Geometry: final body of the model. Coordinates: model frame, mm. Face numbers are marked on the shaded views. Round coordinates to 2 decimals unless told otherwise and drop trailing zeros. Write each loop counter-clockwise with the first axis right and the second up, starting at its lowest first coordinate (ties: lowest second). Pieces come first, ordered by that corner, then holes. Notation, with made-up numbers: (41, 40.5) -> (53, 40.5) arc R22 ccw to (53, 48.5) -> close; hole circle Ø2 at (14.25, -25.75). An arc over 180 degrees is marked (long way). Use one line per item in the form item = value. Start each with the question number.
1. Cut plane A-A, the plane x = 27.5. Return the cut outline in (y, z) (3 decimals).
2. Pin query (flat end, axial travel): pin 1 Ø1.5 at (y, z) = (28.5, 3) entering from -X; pin 2 Ø1.6 at (y, z) = (13.5, 3.5) entering from -X; pin 3 Ø2.5 at (x, z) = (2.5, 2.5) entering from +Y. Return the tip coordinate at first contact, or that it passes through.
3. Cut plane D-D, the plane y = 3.5. Return the cut outline in (x, z).
4. Cut plane B-B, the plane x = 7.5. Return the cut outline in (y, z) (3 decimals), plus the area to 3 significant figures.
5. Draft query along X for the marked faces 1 and 2. Return one class per face: pulls with the +X half, pulls with the -X half, needs draft (parallel to the pull), parting line crosses it, or undercut.
6. Line query: L1, parallel to Y at x = 7.5, z = 1.9 (3 decimals); L2, parallel to Y at x = 8, z = 1.85; L3, parallel to Y at x = 1, z = 3.95. Output: solid intervals per line, ascending.
7. Cut plane C-C, the plane y = 33. Return the cut outline in (x, z), plus the area to 3 significant figures.
```python
from build123d import *

# Parameters (mm, degrees)
SKETCH_1_W           = 40
SKETCH_1_H           = 25
EXTRUDE_1_DEPTH      = 5
SKETCH_2_W           = 25
SKETCH_2_H           = 62
EXTRUDE_2_DEPTH      = 5
SKETCH_3_R           = 8
CUT_EXTRUDE_1_DEPTH  = 14
EXTRUDE_3_DEPTH      = 5
EXTRUDE_4_DEPTH      = 5
SKETCH_6_R           = 1.25
CUT_EXTRUDE_2_DEPTH  = 10
SKETCH_7_R           = 13
CUT_EXTRUDE_3_DEPTH  = 10
FILLET_1_R           = 3
EXTRUDE_6_DEPTH      = 5
FILLET_5_R           = 4
SKETCH_12_R          = 15
SKETCH_12_R_2        = 8
EXTRUDE_7_DEPTH      = 5
CUT_EXTRUDE_6_DEPTH  = 10
SKETCH_14_W          = 30.1
SKETCH_14_H          = 3.1
CUT_EXTRUDE_7_DEPTH  = 5
SKETCH_15_R          = 1.05
CUT_EXTRUDE_8_DEPTH  = 5
SKETCH_18_R          = 1.5
CUT_EXTRUDE_12_DEPTH = 10
SKETCH_20_R          = 1.525
CUT_EXTRUDE_14_DEPTH = 10


with BuildPart() as part:
    # 草图1 → 凸台-拉伸1 (new body)
    with BuildSketch(Plane.XY):
        Rectangle(SKETCH_1_W, SKETCH_1_H)
    extrude(amount=EXTRUDE_1_DEPTH)

    # 草图2 → 凸台-拉伸2 (add)
    with BuildSketch(Plane.XY.offset(5)):
        with Locations((7.5, 43.5)):
            Rectangle(SKETCH_2_W, SKETCH_2_H)
    extrude(amount=-EXTRUDE_2_DEPTH)

    # 草图3 → 切除-拉伸1 (cut)
    with BuildSketch(Plane(origin=(0, 0, 0), x_dir=(-1, 0, 0), z_dir=(0, 0, -1))):
        with Locations((-7.5, 64.5)):
            Circle(SKETCH_3_R)
    extrude(amount=-CUT_EXTRUDE_1_DEPTH, mode=Mode.SUBTRACT)

    # 草图4 → 凸台-拉伸3 (add)
    with BuildSketch(Plane(origin=(0, 0, 0), x_dir=(-1, 0, 0), z_dir=(0, 0, -1))):
        Polygon((5, 74.5), (20, 12.5), (5, 12.5), align=None)
    extrude(amount=-EXTRUDE_3_DEPTH)

    # 草图5 → 凸台-拉伸4 (add)
    with BuildSketch(Plane(origin=(0, 0, 0), x_dir=(-1, 0, 0), z_dir=(0, 0, -1))):
        with BuildLine():
            Line((5, 74.5), (43.961916065, 66.994501049))
            ThreePointArc((43.961916065, 66.994501049), (66.453639267, 36.062373582), (37.102191657, 11.543673671))
            Line((37.102191657, 11.543673671), (20, 12.5))
            Line((20, 12.5), (5, 74.5))
        make_face()
    extrude(amount=-EXTRUDE_4_DEPTH)

    # 草图6 → 切除-拉伸2 (cut)
    with BuildSketch(Plane(origin=(0, 0, 0), x_dir=(-1, 0, 0), z_dir=(0, 0, -1))):
        with Locations((38.665463282, 64)):
            Circle(SKETCH_6_R)
        with Locations((59.883085674, 51.75)):
            Circle(SKETCH_6_R)
        with Locations((59.883085674, 27.25)):
            Circle(SKETCH_6_R)
        with Locations((38.665463282, 15)):
            Circle(SKETCH_6_R)
        with Locations((17.447840889, 27.25)):
            Circle(SKETCH_6_R)
        with Locations((17.447840889, 51.75)):
            Circle(SKETCH_6_R)
    extrude(amount=-CUT_EXTRUDE_2_DEPTH, mode=Mode.SUBTRACT)

    # 草图7 → 切除-拉伸3 (cut)
    with BuildSketch(Plane(origin=(0, 0, 0), x_dir=(-1, 0, 0), z_dir=(0, 0, -1))):
        with Locations((38.665463282, 39.5)):
            Circle(SKETCH_7_R)
    extrude(amount=-CUT_EXTRUDE_3_DEPTH, mode=Mode.SUBTRACT)

    # 圆角1
    fillet_1_edges = [part.edges().sort_by_distance(p)[0] for p in [
        (20, 74.5, 2.5),
        (20, -12.5, 2.5),
        (-20, -12.5, 2.5),
        (-20, 12.5, 2.5),
    ]]
    fillet(fillet_1_edges, radius=FILLET_1_R)

    # 草图9 → 凸台-拉伸6 (add)
    with BuildSketch(Plane(origin=(0, 0, 0), x_dir=(-1, 0, 0), z_dir=(0, 0, -1))):
        Polygon((-17, -12.5), (-35, -12.5), (-35, 12.5), (-19.908611993, 72.234830778), align=None)
    extrude(amount=-EXTRUDE_6_DEPTH)

    # 圆角5
    fillet_5_edges = [part.edges().sort_by_distance(p)[0] for p in [
        (35, -12.5, 2.5),
        (35, 12.5, 2.5),
    ]]
    fillet(fillet_5_edges, radius=FILLET_5_R)

    # 草图12 → 凸台-拉伸7 (add)
    with BuildSketch(Plane(origin=(0, 0, 0), x_dir=(-1, 0, 0), z_dir=(0, 0, -1))):
        with Locations((-7.5, 64.5)):
            Circle(SKETCH_12_R)
        with Locations((-7.5, 64.5)):
            Circle(SKETCH_12_R_2, mode=Mode.SUBTRACT)
    extrude(amount=-EXTRUDE_7_DEPTH)

    # 草图13 → 切除-拉伸6 (cut)
    with BuildSketch(Plane(origin=(0, 0, 0), x_dir=(-1, 0, 0), z_dir=(0, 0, -1))):
        with BuildLine():
            Line((7.401386096, 66.217175707), (7.881923771, 62.047143837))
            ThreePointArc((7.881923771, 62.047143837), (11.961869133, 57.036355872), (18.223004987, 58.633893981))
            ThreePointArc((18.223004987, 58.633893981), (30.76141934, 66.361237674), (45.486790657, 66.65638954))
            Line((45.486790657, 66.65638954), (-3.845717477, 79.048065825))
            ThreePointArc((-3.845717477, 79.048065825), (3.779900034, 74.38756063), (7.401386096, 66.217175707))
        make_face()
    extrude(amount=-CUT_EXTRUDE_6_DEPTH, mode=Mode.SUBTRACT)

    # 草图14 → 切除-拉伸7 (cut)
    with BuildSketch(Plane.XY.offset(5)):
        with Locations((7.5, 14)):
            Rectangle(SKETCH_14_W, SKETCH_14_H)
    extrude(amount=-CUT_EXTRUDE_7_DEPTH, mode=Mode.SUBTRACT)

    # 草图15 → 切除-拉伸8 (cut)
    with BuildSketch(Plane.XY.offset(5)):
        with Locations((-6.5, 15.55)):
            Circle(SKETCH_15_R)
        with Locations((21.5, 15.55)):
            Circle(SKETCH_15_R)
        with Locations((-6.5, 12.45)):
            Circle(SKETCH_15_R)
        with Locations((21.5, 12.45)):
            Circle(SKETCH_15_R)
    extrude(amount=-CUT_EXTRUDE_8_DEPTH, mode=Mode.SUBTRACT)

    # 草图18 → 切除-拉伸12 (cut)
    with BuildSketch(Plane(origin=(0, 0, 0), x_dir=(-1, 0, 0), z_dir=(0, 0, -1))):
        with Locations((-23.5, 0)):
            Circle(SKETCH_18_R)
        with Locations((6.5, 0)):
            Circle(SKETCH_18_R)
    extrude(amount=-CUT_EXTRUDE_12_DEPTH, mode=Mode.SUBTRACT)

    # 草图20 → 切除-拉伸14 (cut)
    with BuildSketch(Plane(origin=(0, 0, 0), x_dir=(-1, 0, 0), z_dir=(0, 0, -1))):
        with Locations((-27.5, 18.5)):
            Circle(SKETCH_20_R)
        with Locations((-7.5, 18.5)):
            Circle(SKETCH_20_R)
    extrude(amount=-CUT_EXTRUDE_14_DEPTH, mode=Mode.SUBTRACT)


solid = part.part
```
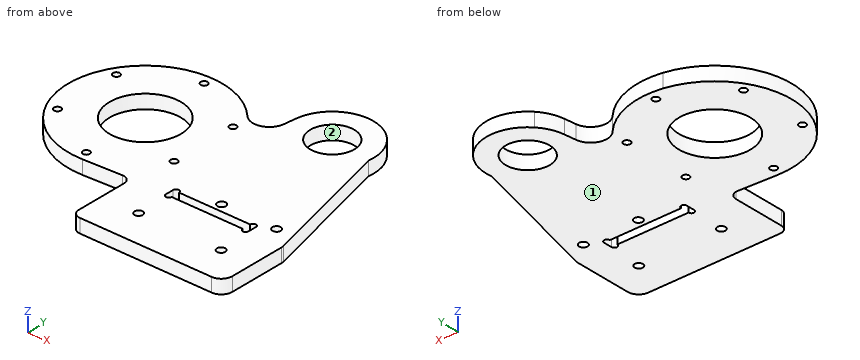
Outcome:
q1.outline = (-12.5, 0) -> (16.975, 0) -> (16.975, 5) -> (-12.5, 5) -> close; (20.025, 0) -> (42.187, 0) -> (42.187, 5) -> (20.025, 5) -> close
q2.pin_1 = -64.72
q2.pin_2 = -50.87
q2.pin_3 = 79.02
q3.outline = (-20, 0) -> (35, 0) -> (35, 5) -> (-20, 5) -> close
q4.outline = (-12.5, 0) -> (12.45, 0) -> (12.45, 5) -> (-12.5, 5) -> close; (15.55, 0) -> (16.975, 0) -> (16.975, 5) -> (15.55, 5) -> close; (20.025, 0) -> (56.5, 0) -> (56.5, 5) -> (20.025, 5) -> close; (72.5, 0) -> (79.5, 0) -> (79.5, 5) -> (72.5, 5) -> close
q4.area = 349 mm^2
q5.face_1 = needs draft
q5.face_2 = undercut
q6.L1 = -12.5 to 12.45, 15.55 to 16.975, 20.025 to 56.5, 72.5 to 79.5
q6.L2 = -12.5 to 12.45, 15.55 to 17.06, 19.94 to 56.52, 72.48 to 79.49
q6.L3 = -12.5 to 12.45, 15.55 to 59.84, 69.16 to 78.02
q7.outline = (-65.9, 0) -> (-49.92, 0) -> (-49.92, 5) -> (-65.9, 5) -> close; (-27.41, 0) -> (29.82, 0) -> (29.82, 5) -> (-27.41, 5) -> close
q7.area = 366 mm^2
